Could you check a few things on this model? Use its own coordinates, in mm. Face numbers are marked on the shaded views. A direction names the side the tool comes from. Give positions to 0.01 mm unless a question says otherwise; leave off trailing zeros. Loops run counter-clockwise (first coordinate to the right, second up) from the corner with the lowest first, then second, coordinate; pieces in that order, holes last.
1. I need wall thicknesses on line 1 along Z through (x, y) = (-4, -400.5); line 2 along Z through (x, y) = (-43.5, -414); line 3 along X through (y, z) = (-472, -109). Which ranges of each line are inside material? Lowest first, please.
2. Imagine slicing it at C-C (x = -14.5). List the corners of the cut face in (y, z) for me.
3. Imagine slicing it at A-A (y = -463). List the corners of the cut face in (x, z) for me.
4. For P1, Ø10, axis at y = -486, z = -59, coming from the +X side; P2, Ø1, axis at x = -50, y = -455.5, coming from the -Z side; P3, Ø8, axis at x = -37, z = -134, coming from the +Y side; P4, Ø4, axis at y = -475.5, z = -118.5, coming from the +X side, each with a flat end and sliding along its axis, tell me the tip position at first contact or that it passes through.
5. For the marked faces 1 and 2, which set-ups out of +Z, -Z, +X, -X, +Y, -Y let a thin tool reach every point of the face, with its end or its side?
6. Imagine slicing it at D-D (y = -409.5). List the corners of the cut face in (x, z) for me.
7. Imagine slicing it at B-B (z = -103.5). List the corners of the cut face in (x, y) for me.
```python
from build123d import *

# Parameters (mm, degrees)
F2_W      = 76.2
F2_H      = 6.35
F2_R      = 2.2225
F3_DEPTH  = 3.175
F6_DEPTH  = 76.2
F8_DEPTH  = 3.175
F11_DEPTH = 3.175


with BuildPart() as f3:
    # F2 (on face) → F3 (new body)
    with BuildSketch(Plane(origin=(29.4081501121, 0, -5.1854503175), x_dir=(0, -1, 0), z_dir=(-0.984807753, 0, 0.1736481777))):
        with Locations((395.4570037365, -172.6052516222)):
            Rectangle(F2_W, F2_H)
        with Locations((370.0570037365, -172.6052516222)):
            Circle(F2_R, mode=Mode.SUBTRACT)
        with Locations((395.4570037365, -172.6052516222)):
            Circle(F2_R, mode=Mode.SUBTRACT)
        with Locations((420.8570037365, -172.6052516222)):
            Circle(F2_R, mode=Mode.SUBTRACT)
    extrude(amount=-F3_DEPTH)

    # F5 (on face) → F6 (join)
    with BuildSketch(Plane.XZ.offset(433.5570037365)):
        Polygon((1.8080008617, -169.4408679692), (-0.0131043237, -172.0416757098), (3.1136602921, -172.5930086739), align=None)
    extrude(amount=-F6_DEPTH)

    # F7 (on face) → F8 (join)
    with BuildSketch(Plane(origin=(-80.8374577566, 0, -115.4478541652), x_dir=(0.8191520443, 0, -0.5735764364), z_dir=(0.5735764364, 0, 0.8191520443))):
        Polygon((98.668316824, -433.5570037365), (98.668316824, -357.3570037365), (-31.963979803, -435.8488063528), (-11.8716898834, -496.0862522298), align=None)
    extrude(amount=F8_DEPTH)

    # F10 (on face) → F11 (join)
    with BuildSketch(Plane(origin=(-207.4110943856, -47.5543564592, -47.6509479128), x_dir=(-0.2125394907, 0.9759316977, -0.0488291537), z_dir=(0.9511529667, 0.2180764118, 0.2185193642))):
        Polygon((-492.3325427071, -31.1929582626), (-459.5935318176, -85.6025820986), (-397.8705177815, -70.6854932975), (-439.3948891587, 0.6603480791), align=None)
    extrude(amount=F11_DEPTH)


solid = f3.part
```
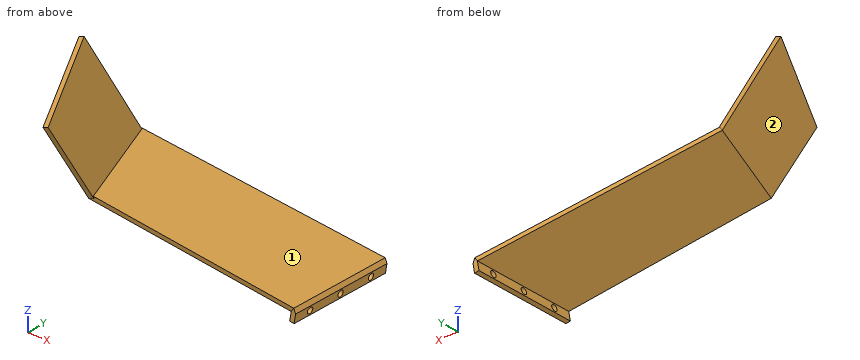
Derived:
1. line 1: z = -169.25 to -165.37
1. line 2: z = -141.59 to -137.72
1. line 3: x = -90.05 to -84.51
2. outline: (-444.82, -158.02) - (-443.56, -161.9) - (-367.98, -161.9) - (-369.32, -158.02) - close
3. outline: (-111.81, -49.17) - (-99.6, -102.31) - (-42.65, -142.19) - (-40.83, -139.59) - (-96.69, -100.47) - (-108.91, -47.25) - close
4. P1: stops at x = -99.32
4. P2: stops at z = -137.39
4. P3: passes through
4. P4: stops at x = -68.09
5. face 1: +Z, +X, +Y
5. face 2: -Z, -X, -Y
6. outline: (-71.1, -122.27) - (-0.01, -172.04) - (-1.12, -178.3) - (2.01, -178.85) - (3.11, -172.59) - (1.81, -169.44) - (-69.28, -119.67) - close
7. outline: (-97.9, -469.23) - (-91.05, -499.09) - (-87.97, -497.99) - (-92.37, -478.81) - (-92.37, -426.43) - (-97.9, -429.16) - close
